Input: part model. Units: mm. Frame: model coordinates. A direction names the side the tool comes from. Coordinates: 2 decimals unless noted, no trailing zeros. Order: outer loops, then holes, each group sorted by start corner. A loop starts at its lowest first (then second) coordinate and runs counter-clockwise, first axis right, second up. Notation, with made-up numbers: M 34.5,-5 L 72.5,-5 A27 ccw 72.5,28 Z; hole C 85,36.25 d3. An arc over 180 degrees is marked long. Answer in a Markdown table with one row per item.
from build123d import *

# Parameters (mm, degrees)
SKETCH_1_R          = 12
EXTRUDE_1_DEPTH     = 4
SKETCH_2_R          = 9.1
CUT_EXTRUDE_1_DEPTH = 3
FILLET_1_R          = 0.5
FILLET_2_R          = 0.5


with BuildPart() as part:
    # 草图1 → 凸台-拉伸1 (new body)
    with BuildSketch(Plane(origin=(0, 0, 0), x_dir=(0, 0, -1), z_dir=(1, 0, 0))):
        Circle(SKETCH_1_R)
    extrude(amount=EXTRUDE_1_DEPTH)

    # 草图2 → 切除-拉伸1 (cut)
    with BuildSketch(Plane(origin=(4, 0, 0), x_dir=(0, 0, -1), z_dir=(1, 0, 0))):
        Circle(SKETCH_2_R)
    extrude(amount=-CUT_EXTRUDE_1_DEPTH, mode=Mode.SUBTRACT)

    # 圆角1
    fillet_1_edges = [part.edges().sort_by_distance(p)[0] for p in [
        (4, 0, 9.1),
    ]]
    fillet(fillet_1_edges, radius=FILLET_1_R)

    # 圆角2
    fillet_2_edges = [part.edges().sort_by_distance(p)[0] for p in [
        (0, 0, 12),
    ]]
    fillet(fillet_2_edges, radius=FILLET_2_R)


solid = part.part
1) Mould query, pull axis Y, two halves, no side actions, for faces 1 (the face through (4, 10, 0)), 2 (the face through (2.23, 0.53, 11.99)), 3 (the face through (1, 0, 0)). Classes: +Y half, -Y half, draft (parallel to the pull), parting line (faces both ways), or undercut.
Resolved:
| item | result |
|---|---|
| face 1 | draft |
| face 2 | parting line |
| face 3 | undercut |
2) Material intervals for probe 1 along Y at (x, z) = (2.4, 0); probe 2 along X at (y, z) = (-4.25, 6.5); probe 3 along Y at (x, z) = (2.55, 5), sorted ascending.
Resolved:
| item | result |
|---|---|
| probe 1 | y = -12 to -9.1, 9.1 to 12 |
| probe 2 | x = 0 to 1 |
| probe 3 | y = -10.91 to -7.6, 7.6 to 10.91 |
3) Contact query for flat-ended pins moving along their axis: pin 1 (1.5 mm diameter, centred on y = 7, z = 1.5, fed in from -X); pin 2 (1.5 mm diameter, centred on y = 7, z = -3, fed in from +X); pin 3 (1 mm diameter, centred on x = 2.5, z = -3, fed in from +Y); pin 4 (1 mm diameter, centred on x = 3, y = -7, fed in from -Z). Output: stop coordinate, or through.
Resolved:
| item | result |
|---|---|
| pin 1 | stops at x = 0 |
| pin 2 | stops at x = 1 |
| pin 3 | stops at y = 11.74 |
| pin 4 | stops at z = -10.09 |
4) Cut plane C-C, the plane x = 1.8. Output: boundary loops of the cut face in (y, z).
Resolved:
| item | result |
|---|---|
| outline | C 0,0 d24; hole C 0,0 d18.2 |
5) Reachability of faces 4 (the face through (2.268, -8.884, 1.973)), 5 (the face through (0, 0, 0)) from +Z, -Z, +X, -X, +Y, -Y: full face, straight path, thin tool, end or side. Return the list, or none.
Resolved:
| item | result |
|---|---|
| face 4 | +X |
| face 5 | +Z, -Z, -X, +Y, -Y |
6) Cut plane A-A, the plane z = 0. Output: boundary loops of the cut face in (x, y), and give its area (3 significant figures).
Resolved:
| item | result |
|---|---|
| outline | M 0,-11.5 A0.5 ccw 0.5,-12 L 4,-12 L 4,-9.6 A0.5 ccw 3.5,-9.1 L 1,-9.1 L 1,9.1 L 3.5,9.1 A0.5 ccw 4,9.6 L 4,12 L 0.5,12 A0.5 ccw 0,11.5 Z |
| area | 41.2 mm2 |
